```python
from build123d import *

# Parameters (mm, degrees)
BOSS_EXTRUDE1_DEPTH = 6.35
CUT_EXTRUDE1_DEPTH  = 194.156212688
SKETCH5_R           = 1.5
CUT_EXTRUDE2_DEPTH  = 155.564945897
FILLET1_R           = 30
CHAMFER1_SIZE       = 5
FILLET2_R           = 5
FILLET3_R           = 5
SKETCH6_W           = 7
SKETCH6_H           = 10
CUT_EXTRUDE3_DEPTH  = 194.156212688
HOLE1_D             = 4.4
HOLE1_CBORE_D       = 7.5
HOLE1_CBORE_DEPTH   = 3
HOLE2_D             = 4.4
HOLE2_CBORE_D       = 7.5
HOLE2_CBORE_DEPTH   = 3
FILLET4_R           = 5
HOLE3_D             = 4.4
HOLE3_CBORE_D       = 7.5
HOLE3_CBORE_DEPTH   = 3


with BuildPart() as part:
    # Sketch1 → Boss-Extrude1 (new body)
    with BuildSketch(Plane.XY):
        Polygon((0, 0), (-138, 0), (-138, 30), (-63, 30), (-63, 40), (-138, 40), (-138, 59), (-112, 59), (-112, 87), (-90, 87), (-90, 135), (0, 135), align=None)
    extrude(amount=BOSS_EXTRUDE1_DEPTH)

    # Sketch4 → Cut-Extrude1 (cut, through all)
    with BuildSketch(Plane(origin=(0, 0, 0), x_dir=(-1, 0, 0), z_dir=(0, 0, -1))):
        Polygon((120, 40), (138, 45), (138, 40), align=None)
        Polygon((120, 30), (138, 30), (138, 25), align=None)
    extrude(amount=-CUT_EXTRUDE1_DEPTH, mode=Mode.SUBTRACT)

    # Sketch5 → Cut-Extrude2 (cut, through all)
    with BuildSketch(Plane.ZY.offset(63)):
        with Locations((3.175, 35)):
            Circle(SKETCH5_R)
    extrude(amount=-CUT_EXTRUDE2_DEPTH, mode=Mode.SUBTRACT)

    # Fillet1
    fillet1_edges = [part.edges().sort_by_distance(p)[0] for p in [
        (-120, 40, 3.175),
        (-120, 30, 3.175),
    ]]
    fillet(fillet1_edges, radius=FILLET1_R)

    # Chamfer1
    chamfer1_edges = [part.edges().sort_by_distance(p)[0] for p in [
        (-90, 111, 6.35),
        (-112, 73, 6.35),
    ]]
    chamfer(chamfer1_edges, length=CHAMFER1_SIZE)

    # Fillet2
    fillet2_edges = [part.edges().sort_by_distance(p)[0] for p in [
        (-138, 59, 3.175),
        (-138, 45, 3.175),
        (-138, 25, 3.175),
    ]]
    fillet(fillet2_edges, radius=FILLET2_R)

    # Fillet3
    fillet3_edges = [part.edges().sort_by_distance(p)[0] for p in [
        (-112, 59, 0.675),
        (-90, 87, 0.675),
        (-109.5, 59, 3.85),
        (-87.5, 87, 3.85),
    ]]
    fillet(fillet3_edges, radius=FILLET3_R)

    # Sketch6 → Cut-Extrude3 (cut, through all)
    with BuildSketch(Plane(origin=(0, 0, 0), x_dir=(-1, 0, 0), z_dir=(0, 0, -1))):
        with Locations((3.5, 35)):
            Rectangle(SKETCH6_W, SKETCH6_H)
    extrude(amount=-CUT_EXTRUDE3_DEPTH, mode=Mode.SUBTRACT)

    # Hole1 (through all)
    with Locations(Plane(origin=(0, 0, 0), x_dir=(-1, 0, 0), z_dir=(0, 0, -1))):
        with Locations((3.175, 125), (3.175, 67.5), (3.175, 10)):
            CounterBoreHole(HOLE1_D / 2, HOLE1_CBORE_D / 2, HOLE1_CBORE_DEPTH)

    # Hole2 (through all)
    with Locations(Plane(origin=(0, 0, 0), x_dir=(-1, 0, 0), z_dir=(0, 0, -1))):
        with Locations((17.4, 117), (17.4, 80), (17.4, 28)):
            CounterBoreHole(HOLE2_D / 2, HOLE2_CBORE_D / 2, HOLE2_CBORE_DEPTH)

    # Fillet4
    fillet4_edges = [part.edges().sort_by_distance(p)[0] for p in [
        (-109.5, 87, 3.85),
    ]]
    fillet(fillet4_edges, radius=FILLET4_R)

    # Hole3 (through all)
    with Locations(Plane(origin=(0, 0, 0), x_dir=(-1, 0, 0), z_dir=(0, 0, -1))):
        with Locations((87.870353785, 4.293591352), (114.451398707, 7.906888356), (130.844995532, 4.293591352)):
            CounterBoreHole(HOLE3_D / 2, HOLE3_CBORE_D / 2, HOLE3_CBORE_DEPTH)


solid = part.part
```
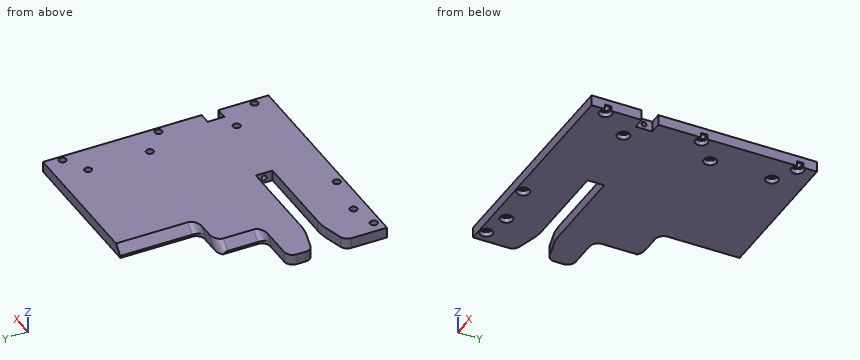
Work out the finished part from the listing and answer in its coordinate system (mm). Coordinates: 2 decimals unless noted, no trailing zeros. Loops run counter-clockwise (first coordinate to the right, second up) from the corner with the lowest first, then second, coordinate; pieces in that order, holes last. Notation, with made-up numbers: M 31.25,-26 L 74.25,-26 A29 ccw 74.25,10 Z; hole C 25.25,49.5 d5. An arc over 180 degrees is marked long. Use CSV: the item, a comma, the result in double quotes. Start each with the question number.
(1) Find section C-C, the plane y = 96. Give the vertices of the cut face in (x, z), then the cut area to 3 significant figures.
(2) Find section A-A, the plane y = 125. Give the vertices of the cut face in (x, z) (3 decimals).
(3) Find section B-B, the plane x = -121. Give the vertices of the cut face in (y, z).
(4) Consider line 1 (Y direction, x = -75, z = 3.75); line 2 (Y direction, x = -11, z = 3.5); line 3 (Y direction, x = -17.4, z = 1.8). Determine where each line is inside the solid, lowest interval first.
(5) Given pin 1 Ø3.5 at (x, y) = (-3.175, 125) entering from -Z; pin 2 Ø7 at (x, y) = (-17.4, 80) entering from -Z; pin 3 Ø0.7 at (y, z) = (76.5, 0.5) entering from -X; pin 4 Ø2 at (y, z) = (101, 4.5) entering from -X, each flat-ended and moving along its own axis, determine where each tip first touches the part or whether it passes through.
Recorded:
1,outline,"M -90,0 L 0,0 L 0,6.35 L -85,6.35 L -90,1.35 Z"
1,area,"559 mm^2"
2,outline,"M -90,0 L -6.925,0 L -6.925,3 L -5.375,3 L -5.375,6.35 L -85,6.35 L -90,1.35 Z; M -0.975,3 L 0,3 L 0,6.35 L -0.975,6.35 Z"
3,outline,"M 0,0 L 29.57,0 L 29.57,6.35 L 0,6.35 Z; M 40.43,0 L 59,0 L 59,6.35 L 40.43,6.35 Z"
4,line 1,"y = 0 to 30, 40 to 135"
4,line 2,"y = 0 to 33.54, 36.46 to 135"
4,line 3,"y = 0 to 24.25, 31.75 to 34.4, 35.6 to 76.25, 83.75 to 113.25, 120.75 to 135"
5,pin 1,"passes through"
5,pin 2,"stops at z = 3"
5,pin 3,"stops at x = -112"
5,pin 4,"stops at x = -87.85"
